For this review, take the finished solid that the model builds, in its own axes (mm). Face numbers are marked on the shaded views. A direction names the side the tool comes from. Give positions to 0.01 mm unless a question says otherwise; leave off trailing zeros. Order: outer loops, then holes, each group sorted by start corner. A loop starts at its lowest first (then second) coordinate and runs counter-clockwise, first axis right, second up. Notation, with made-up numbers: (31.25, -6) - (43.25, -6) arc R21 cw to (43.25, 19) - close; hole circle Ø4 at (84, -11.75). An arc over 180 degrees is marked (long way). Answer as a JSON object with one key per item and string values. Group by question number.
from build123d import *

# Parameters (mm, degrees)
BOSS_EXTRUDE1_DEPTH      = 5
BOSS_EXTRUDE1_DEPTH_BACK = 34
SKETCH1_R                = 18
SKETCH2_R                = 14
BOSS_EXTRUDE2_DEPTH      = 50
BOSS_EXTRUDE3_START      = 80
SKETCH3_R                = 14
BOSS_EXTRUDE3_DEPTH      = 80
CUT_EXTRUDE2_DEPTH       = 9
SKETCH6_R                = 19.5
SKETCH6_R_2              = 18
BOSS_EXTRUDE4_DEPTH      = 4
SKETCH10_R               = 19.5
SKETCH10_R_2             = 18
BOSS_EXTRUDE6_DEPTH      = 1.5
SKETCH12_W               = 2.4
SKETCH12_H               = 5.371583629
SKETCH13_R               = 18
BOSS_EXTRUDE7_DEPTH      = 2
SKETCH14_W               = 5.5
SKETCH14_H               = 45
SKETCH17_R               = 14.891727411
CUT_EXTRUDE4_DEPTH       = 18
BOSS_EXTRUDE8_START      = 3
SKETCH18_R               = 14
BOSS_EXTRUDE8_DEPTH      = 3
SKETCH19_R               = 18
BOSS_EXTRUDE9_DEPTH      = 26
SKETCH20_R               = 17.17468577
SKETCH20_R_2             = 9.25
CUT_EXTRUDE5_DEPTH       = 6
BOSS_EXTRUDE10_START     = 40
SKETCH21_R               = 9.25
BOSS_EXTRUDE10_DEPTH     = 40
SKETCH22_R               = 12
BOSS_EXTRUDE11_DEPTH     = 4
CHAMFER1_SIZE            = 1
CUT_EXTRUDE6_DEPTH       = 10


with BuildPart() as part:
    # Sketch1 → Boss-Extrude1 (new, two sides: drawn at the far end of the back side and taken through both)
    with BuildSketch(Plane.XY.offset(-BOSS_EXTRUDE1_DEPTH_BACK)):
        Circle(SKETCH1_R)
    extrude(amount=BOSS_EXTRUDE1_DEPTH + BOSS_EXTRUDE1_DEPTH_BACK)

    # Sketch2 → Boss-Extrude2 (add)
    with BuildSketch(Plane.XY.offset(5)):
        Circle(SKETCH2_R)
    extrude(amount=BOSS_EXTRUDE2_DEPTH)

    # Sketch3 → Boss-Extrude3 (add)
    with BuildSketch(Plane(origin=(0, 0, -34), x_dir=(-1, 0, 0), z_dir=(0, 0, -1)).offset(BOSS_EXTRUDE3_START)):
        with Locations(Location((0, 0, 0), (0, 0, 180))):
            Circle(SKETCH3_R)
    extrude(amount=-BOSS_EXTRUDE3_DEPTH)

    # Sketch5 → Cut-Extrude2 (cut)
    with BuildSketch(Plane.XZ.offset(-21.3)):
        with BuildLine():
            Line((-5, -5), (-5, -22))
            ThreePointArc((-5, -22), (0, -27), (5, -22))
            Line((5, -22), (5, -5))
            ThreePointArc((5, -5), (0, 0), (-5, -5))
        make_face()
    extrude(amount=CUT_EXTRUDE2_DEPTH, mode=Mode.SUBTRACT)

    # Sketch6 → Boss-Extrude4 (add)
    with BuildSketch(Plane(origin=(0, 0, -34), x_dir=(-1, 0, 0), z_dir=(0, 0, -1))):
        Circle(SKETCH6_R)
        with Locations(Location((0, 0, 0), (0, 0, 270))):
            Circle(SKETCH6_R_2, mode=Mode.SUBTRACT)
    extrude(amount=-BOSS_EXTRUDE4_DEPTH)

    # Sketch10 → Boss-Extrude6 (add)
    with BuildSketch(Plane.XY.offset(-30)):
        with Locations(Location((0, 0, 0), (0, 0, 180))):
            Circle(SKETCH10_R)
        Circle(SKETCH10_R_2, mode=Mode.SUBTRACT)
    extrude(amount=BOSS_EXTRUDE6_DEPTH)

    # Sketch12 → Cut-Revolve1 (revolve, cut)
    with BuildSketch(Plane(origin=(0, 0, 0), x_dir=(0, 0, -1), z_dir=(1, 0, 0)), mode=Mode.PRIVATE) as cut_revolve1_sk:
        with Locations((-2.7, 19.085791815)):
            Rectangle(SKETCH12_W, SKETCH12_H)
    revolve(cut_revolve1_sk.sketch.rotate(Axis((0, 0, 1.5), (0, 0, -1)), 90), axis=Axis((0, 0, 1.5), (0, 0, -1)), mode=Mode.SUBTRACT)

    # Sketch13 → Boss-Extrude7 (add)
    with BuildSketch(Plane.XY.offset(5)):
        Circle(SKETCH13_R)
    extrude(amount=BOSS_EXTRUDE7_DEPTH)

    # Sketch14 → Revolve1 (revolve)
    with BuildSketch(Plane(origin=(0, 0, 0), x_dir=(1, 0, 0), z_dir=(0, 1, 0)), mode=Mode.PRIVATE) as revolve1_sk:
        with Locations((16.75, 56.5)):
            Rectangle(SKETCH14_W, SKETCH14_H)
    revolve(revolve1_sk.sketch.rotate(Axis((0, 0, -114), (0, 0, 1)), 180), axis=Axis((0, 0, -114), (0, 0, 1)))

    # Sketch17 → Cut-Extrude4 (cut)
    with BuildSketch(Plane(origin=(0, 0, -114), x_dir=(-1, 0, 0), z_dir=(0, 0, -1))):
        Circle(SKETCH17_R)
    extrude(amount=-CUT_EXTRUDE4_DEPTH, mode=Mode.SUBTRACT)

    # Sketch18 → Boss-Extrude8 (add)
    with BuildSketch(Plane(origin=(0, 0, -96), x_dir=(-1, 0, 0), z_dir=(0, 0, -1)).offset(BOSS_EXTRUDE8_START)):
        with Locations(Location((0, 0, 0), (0, 0, 180))):
            Circle(SKETCH18_R)
    extrude(amount=-BOSS_EXTRUDE8_DEPTH)

    # Sketch19 → Boss-Extrude9 (add)
    with BuildSketch(Plane.XY.offset(7)):
        Circle(SKETCH19_R)
    extrude(amount=BOSS_EXTRUDE9_DEPTH)

    # Sketch20 → Cut-Extrude5 (cut)
    with BuildSketch(Plane.XY.offset(55)):
        Circle(SKETCH20_R)
        Circle(SKETCH20_R_2, mode=Mode.SUBTRACT)
    extrude(amount=-CUT_EXTRUDE5_DEPTH, mode=Mode.SUBTRACT)

    # Sketch21 → Boss-Extrude10 (add)
    with BuildSketch(Plane.XY.offset(55).offset(BOSS_EXTRUDE10_START)):
        Circle(SKETCH21_R)
    extrude(amount=-BOSS_EXTRUDE10_DEPTH)

    # Sketch22 → Boss-Extrude11 (add)
    with BuildSketch(Plane.XY.offset(49)):
        Circle(SKETCH22_R)
    extrude(amount=BOSS_EXTRUDE11_DEPTH)

    # Chamfer1
    chamfer1_edges = [part.edges().sort_by_distance(p)[0] for p in [
        (-14, 0, -99),
        (-9.25, 0, 95),
    ]]
    chamfer(chamfer1_edges, length=CHAMFER1_SIZE)

    # Sketch24 → Cut-Extrude6 (cut)
    with BuildSketch(Plane(origin=(0, 6, 0), x_dir=(1, 0, 0), z_dir=(0, 1, 0))):
        with BuildLine():
            Line((3, -70), (3, -85))
            ThreePointArc((3, -85), (0, -88), (-3, -85))
            Line((-3, -85), (-3, -70))
            ThreePointArc((-3, -70), (0, -67), (3, -70))
        make_face()
    extrude(amount=CUT_EXTRUDE6_DEPTH, mode=Mode.SUBTRACT)


solid = part.part
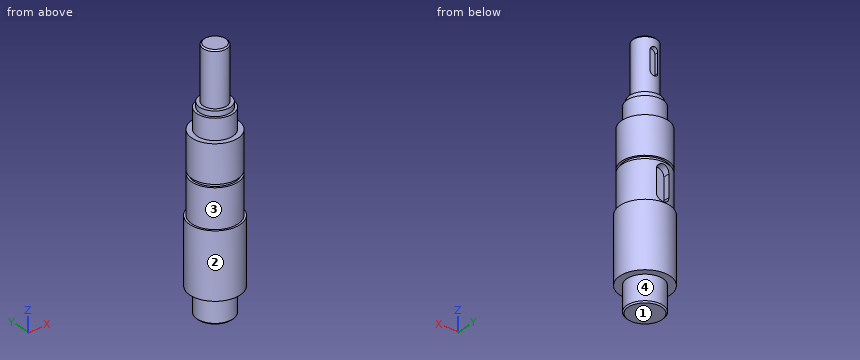
1) For line 1 (Z direction, x = 15, y = -9.5); line 2 (Z direction, x = 0, y = -15.5); line 3 (Y direction, x = -0.5, z = -75), list the stretches that pass through material, from the lowest coordinate up.
2) For pin 1 (1.4 mm diameter, centred on y = 7, z = 76, fed in from -X); pin 2 (10 mm diameter, centred on x = -1, z = 23.5, fed in from +Y); pin 3 (5 mm diameter, centred on x = 12.5, z = 44.5, fed in from +Y), all flat-tipped, find the tip position at first contact; note any pin that passes through.
3) Consider section B-B (z = -18). Give the boundary of the cut face in (x, y).
4) Consider section C-C (z = 7.5). Give the boundary of the cut face in (x, y).
5) For the marked faces 3 and 4, list the 3-axis set-ups (+Z, -Z, +X, -X, +Y, -Y) from which the entire face can be reached by the end or side of a thin tool; tool diameter is ignored.
6) Mouldability with a two-part tool opening along Z and no side actions: class the marked faces 1 and 2 as released by +Z, released by -Z, zero draft, split by the parting line, or undercut.
7) Consider section A-A (z = 72). Give the boundary of the cut face in (x, y).
Result set:
{
 "1": {"line 1": "z = -79 to 1.5, 3.9 to 33", "line 2": "z = -79 to 33", "line 3": "y = -19.49 to 19.49"},
 "2": {"pin 1": "stops at x = -6.77", "pin 2": "stops at y = 18", "pin 3": "stops at y = 9.8"},
 "3": {"outline": "(-5, 12.3) - (-5, 17.29) arc R18 ccw (long way) to (5, 17.29) - (5, 12.3) - close"},
 "4": {"outline": "circle Ø36 at (0, 0)"},
 "5": {"face 3": "+Z", "face 4": "-Z"},
 "6": {"face 1": "released by -Z", "face 2": "zero draft"},
 "7": {"outline": "(-3, 6) - (-3, 8.75) arc R9.25 ccw (long way) to (3, 8.75) - (3, 6) - close"}
}
